```python
from build123d import *

# Parameters (mm, degrees)
SKETCH1_R           = 24.5
SKETCH1_R_2         = 21
BOSS_EXTRUDE1_DEPTH = 130
SKETCH3_R           = 24.5
SKETCH3_R_2         = 21
BOSS_EXTRUDE2_DEPTH = 65


with BuildPart() as part:
    # Sketch1 → Boss-Extrude1 (new body)
    with BuildSketch(Plane(origin=(0, 0, 0), x_dir=(1, 0, 0), z_dir=(0, 1, 0))):
        Circle(SKETCH1_R)
        Circle(SKETCH1_R_2, mode=Mode.SUBTRACT)
    extrude(amount=BOSS_EXTRUDE1_DEPTH)

    # Sketch3 → Boss-Extrude2 (add)
    with BuildSketch(Plane.XY):
        with Locations((0, 65)):
            Circle(SKETCH3_R)
        with Locations((0, 65)):
            Circle(SKETCH3_R_2, mode=Mode.SUBTRACT)
    extrude(amount=BOSS_EXTRUDE2_DEPTH)


solid = part.part
```
Can you work these out from the model? Positions are in its coordinate system, mm. A direction names the side the tool comes from. Give positions to 0.01 mm unless a question says otherwise; leave off trailing zeros. Write each loop counter-clockwise with the first axis right and the second up, starting at its lowest first coordinate (ties: lowest second). Pieces come first, ordered by that corner, then holes. Notation, with made-up numbers: (77, 23) - (99, 23) arc R17 ccw to (99, 50) - close; hole circle Ø2 at (2, -30). An arc over 180 degrees is marked (long way). Write item = value, one per line. Start each with the question number.
1. Imagine slicing it at D-D (x = -6). Please give me the cut outline in (y, z).
2. Please list where these lines run through material, in increasing order: line 1 (Y direction, x = -1, z = 19); line 2 (X direction, y = 65, z = 47); line 3 (X direction, y = 83, z = 9.5).
3. For pin 1 (1.5 mm diameter, centred on x = 12, y = 95.5, fed in from +Z); pin 2 (25 mm diameter, centred on x = 0, y = 65, fed in from -Z); pin 3 (1 mm diameter, centred on y = 72, z = 44, fed in from +X), each with a flat end and sliding along its axis, tell me the tip position at first contact or that it passes through.
4. On a 3-axis mill with a long thin cutter (end or side, diameter ignored), from which of +Z, -Z, +X, -X, +Y, -Y can I reach the whole of each face in a straight line? I mean faces 1 (the face through (20, 72, 65)), 2 (the face through (20.03, 71.31, 44.26)), 3 (the face through (0, 44, 8)). Say none if no direction works.
5. Imagine slicing it at C-C (z = 28.5). Please give me the cut outline in (x, y).
6. Imagine slicing it at B-B (y = 59). Please give me the cut outline in (x, z).
7. Imagine slicing it at A-A (x = 0). Please give me the cut outline in (y, z).
8. Thinking about a two-plate mould opening in Z: for faces 4 (the face through (-1.7, 86.4, 0)), 5 (the face through (20, 130, -7)), 6 (the face through (-3.19, 64.09, -24.29)), which applies, released by +Z, released by -Z, zero draft, split by the parting line, or undercut?
Worked answers:
q1.outline = (0, -23.75) - (130, -23.75) - (130, -20.12) - (0, -20.12) - close; (0, 20.12) - (41.25, 20.12) - (41.25, 0) - (44.88, 0) - (44.88, 20.12) - (85.12, 20.12) - (85.12, 0) - (88.75, 0) - (88.75, 20.12) - (130, 20.12) - (130, 23.75) - (88.75, 23.75) - (88.75, 65) - (85.12, 65) - (85.12, 23.75) - (44.88, 23.75) - (44.88, 65) - (41.25, 65) - (41.25, 23.75) - (0, 23.75) - close
q2.line_1 = 40.52 to 44.02, 85.98 to 89.48
q2.line_2 = -24.5 to -21, 21 to 24.5
q2.line_3 = -22.58 to -18.73, -16.62 to -10.82, 10.82 to 16.62, 18.73 to 22.58
q3.pin_1 = 21.76
q3.pin_2 = -24.5
q3.pin_3 = 23.62
q4.face_1 = +Z, +X, -X, +Y, -Y
q4.face_2 = +Z
q4.face_3 = none
q5.outline = circle Ø49 at (0, 65); hole circle Ø42 at (0, 65)
q6.outline = (-23.75, 6) arc R24.5 ccw (long way) to (23.75, 6) - (23.75, 65) - (20.12, 65) - (20.12, 13.97) arc R24.5 ccw to (-20.12, 13.97) - (-20.12, 65) - (-23.75, 65) - close; hole (-21, 0) arc R21 ccw to (21, 0) - (20.12, 0) - (20.12, 6) arc R21 ccw to (-20.12, 6) - (-20.12, 0) - close
q7.outline = (0, -24.5) - (130, -24.5) - (130, -21) - (0, -21) - close; (0, 21) - (40.5, 21) - (40.5, 0) - (44, 0) - (44, 21) - (86, 21) - (86, 0) - (89.5, 0) - (89.5, 21) - (130, 21) - (130, 24.5) - (89.5, 24.5) - (89.5, 65) - (86, 65) - (86, 24.5) - (44, 24.5) - (44, 65) - (40.5, 65) - (40.5, 24.5) - (0, 24.5) - close
q8.face_4 = undercut
q8.face_5 = zero draft
q8.face_6 = split by the parting line
